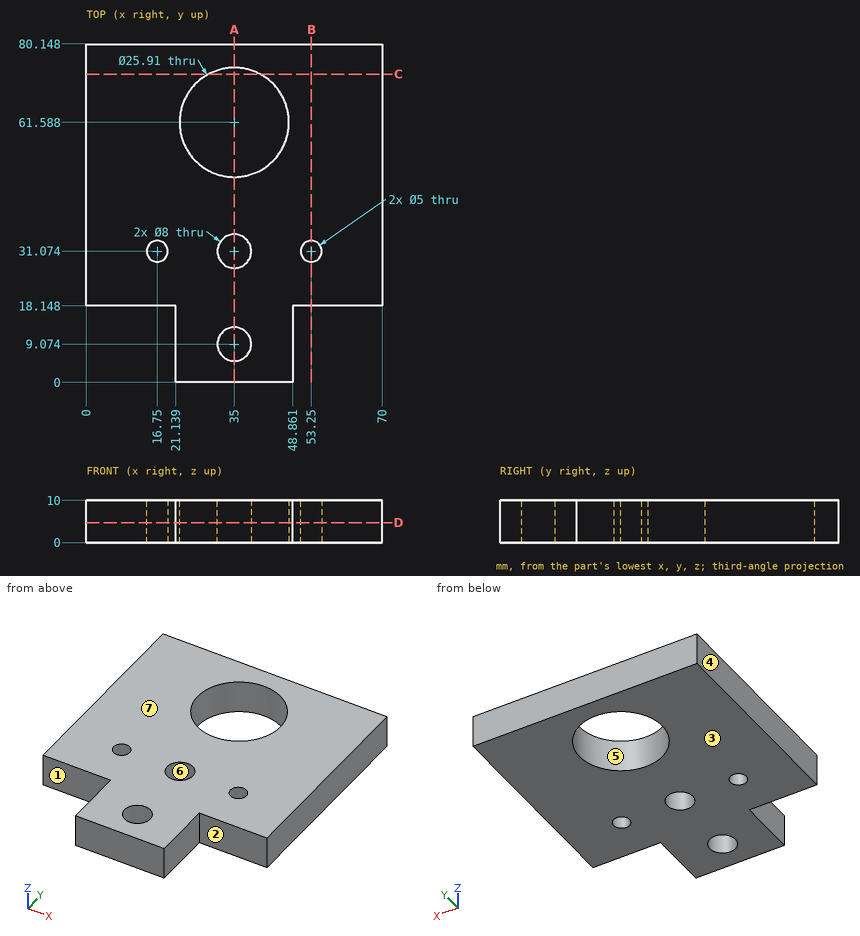
Could you check a few things on this drawing? It's one solid part, dimensions in mm from its lowest x, y, z. A direction names the side the tool comes from. Coordinates: 2 decimals unless noted, no trailing zeros. Order: outer loops, then holes, each group sorted by start corner. A loop starts at its lowest first (then second) coordinate and runs counter-clockwise, first axis right, second up. Notation, with made-up numbers: M -27.5,-28 L 1.5,-28 A34 cw 1.5,8 Z; hole C -27,23.5 d4. An arc over 180 degrees is marked long. Answer as a JSON object with one key per item and string values. Group by question number.
(1) For pin 1 (3 mm diameter, centred on x = 58, z = 7.5, fed in from -Y); pin 2 (5 mm diameter, centred on y = 10, z = 5, fed in from -X), each with a flat end and sliding along its axis, tell me the tip position at first contact or that it passes through.
(2) Suppose I cut it at A-A, the plane x = 35. Please give me the cut outline in (y, z).
(3) Suppose I cut it at D-D, the plane z = 4.75. State how many separate pieces and enclosed holes the cut face has, then the cut area to 3 significant figures.
(4) Suppose I cut it at B-B, the plane x = 53.25. Please give me the cut outline in (y, z).
(5) I need wall thicknesses on probe 1 along Y at (x, z) = (35, 5.25); probe 2 along X at (y, z) = (61, 9.25); probe 3 along Y at (x, z) = (38, 6) (1 decimal). Which ranges of each line are inside material? Lowest first, please.
(6) Which directions (+Z, -Z, +X, -X, +Y, -Y) give clear straight access to the entire face, cutting with the end or side of a thin tool? Please do the marked faces 1, 2 and 3.
(7) If we mould it in two halves opening along X, with no side actions, what happens to the marked faces 4, 5, 6 and 7? For each: released by +X, released by -X, zero draft, split by the parting line, or undercut.
(8) Suppose I cut it at C-C, the plane y = 73. Please give me the cut outline in (x, z).
Values found:
{
 "1": {"pin 1": "stops at y = 18.15", "pin 2": "stops at x = 21.14"},
 "2": {"outline": "M 0,0 L 5.07,0 L 5.07,10 L 0,10 Z; M 13.07,0 L 27.07,0 L 27.07,10 L 13.07,10 Z; M 35.07,0 L 48.63,0 L 48.63,10 L 35.07,10 Z; M 74.54,0 L 80.15,0 L 80.15,10 L 74.54,10 Z"},
 "3": {"separate pieces": "1", "enclosed holes": "5", "area": "4,180 mm^2"},
 "4": {"outline": "M 18.15,0 L 28.57,0 L 28.57,10 L 18.15,10 Z; M 33.57,0 L 80.15,0 L 80.15,10 L 33.57,10 Z"},
 "5": {"probe 1": "y = 0 to 5.07, 13.07 to 27.07, 35.07 to 48.63, 74.54 to 80.15", "probe 2": "x = 0 to 22.06, 47.94 to 70", "probe 3": "y = 0 to 6.4, 11.7 to 28.4, 33.7 to 49, 74.2 to 80.1"},
 "6": {"face 1": "+Z, -Z, -X, -Y", "face 2": "+Z, -Z, +X, -Y", "face 3": "-Z, +X, -X, +Y, -Y"},
 "7": {"face 4": "released by -X", "face 5": "undercut", "face 6": "undercut", "face 7": "zero draft"},
 "8": {"outline": "M 0,0 L 28.87,0 L 28.87,10 L 0,10 Z; M 41.13,0 L 70,0 L 70,10 L 41.13,10 Z"}
}
